Read the model definition and answer for the solid it produces. Units are mm, in the model's axes. Coordinates: 2 decimals unless noted, no trailing zeros. Loops run counter-clockwise (first coordinate to the right, second up) from the corner with the lowest first, then second, coordinate; pieces in that order, holes last. Notation, with made-up numbers: (-3, 79) -> (39, 79) arc R27 ccw to (39, 103) -> close; hole circle Ø10 at (51, 5). An arc over 180 degrees is marked (long way). Answer as a JSON object with one key per item and string values. Group by question number.
1) Determine the mould class of faces 1 (the face through (2.348, 0.628, 14.274)), 2 (the face through (2.3, 41.5, 5.6)), 3 (the face through (2.35, 46.52, -0.54)), 4 (the face through (0, 23, 5)) for opening direction Y: released by +Y, released by -Y, zero draft, split by the parting line, or undercut.
2) Consider probe 1 along Y at (x, z) = (3.25, 7.5); probe 2 along Z at (x, y) = (2.6, -0.5); probe 3 along Z at (x, y) = (4.2, -7.5). Determine where each line is inside the solid, lowest interval first. Write a range as [from, to].
3) Section A-A, the plane x = 2.7 is taken. Count the separate pieces of the cut face and the enclosed holes in it, plus the area to 3 significant figures.
4) Section B-B, the plane y = 38.1 is taken. Give the vertices of the cut face in (x, z), plus the area to 3 significant figures.
5) A flat-ended cylindrical pin translates along its axis: P1, Ø5.5, axis at y = 38.1, z = 5.14, coming from the +X side. Find the tip coordinate at first contact, or state that the pin passes through.
6) Section C-C, the plane y = -12 is taken. Give the vertices of the cut face in (x, z), plus the area to 3 significant figures.
7) Section D-D, the plane z = 0 is taken. Give the vertices of the cut face in (x, y).
from build123d import *

# Parameters (mm, degrees)
SKETCH1_R           = 14.2875
SKETCH1_R_2         = 3.429
BOSS_EXTRUDE1_DEPTH = 4.7625


with BuildPart() as part:
    # Sketch1 → Boss-Extrude1 (new body)
    with BuildSketch(Plane(origin=(0, 0, 0), x_dir=(0, 0, -1), z_dir=(1, 0, 0))):
        with BuildLine():
            Line((-20.3835, 48.26), (-5.1435, 48.26))
            ThreePointArc((-5.1435, 48.26), (0.606928002, 46.476047862), (4.337968538, 41.750664919))
            Line((4.337968538, 41.750664919), (17.77775351, 6.844996724))
            ThreePointArc((17.77775351, 6.844996724), (6.097008594, -18.047963492), (-18.286717832, -5.33839404))
            Line((-18.286717832, -5.33839404), (-30.136416177, 35.252856512))
            ThreePointArc((-30.136416177, 35.252856512), (-28.512232307, 44.195023468), (-20.3835, 48.26))
        make_face()
        Circle(SKETCH1_R, mode=Mode.SUBTRACT)
        with Locations((-20.3835, 38.1)):
            Circle(SKETCH1_R_2, mode=Mode.SUBTRACT)
        with Locations((-5.1435, 38.1)):
            Circle(SKETCH1_R_2, mode=Mode.SUBTRACT)
    extrude(amount=BOSS_EXTRUDE1_DEPTH)


solid = part.part
Determined:
{
 "1": {"face 1": "undercut", "face 2": "undercut", "face 3": "released by +Y", "face 4": "zero draft"},
 "2": {"probe 1": "[-17.51, -12.16], [12.16, 35.61], [40.59, 48.26]", "probe 2": "[-19.04, -14.28], [14.28, 19.7]", "probe 3": "[-17.51, -12.16], [12.16, 17.51]"},
 "3": {"separate pieces": "1", "enclosed holes": "3", "area": "1,640 mm²"},
 "4": {"outline": "(0, -5.74) -> (4.76, -5.74) -> (4.76, 1.71) -> (0, 1.71) -> close; (0, 8.57) -> (4.76, 8.57) -> (4.76, 16.95) -> (0, 16.95) -> close; (0, 23.81) -> (4.76, 23.81) -> (4.76, 30.54) -> (0, 30.54) -> close", "area": "107 mm²"},
 "5": {"P1": "through"},
 "6": {"outline": "(0, -14.8) -> (4.76, -14.8) -> (4.76, -7.75) -> (0, -7.75) -> close; (0, 7.75) -> (4.76, 7.75) -> (4.76, 14.8) -> (0, 14.8) -> close", "area": "67.1 mm²"},
 "7": {"outline": "(0, -19.05) -> (4.76, -19.05) -> (4.76, -14.29) -> (0, -14.29) -> close; (0, 14.29) -> (4.76, 14.29) -> (4.76, 46.86) -> (0, 46.86) -> close"}
}
